Here's the drawing with two shaded views (mm, measured from the low corner). I have some questions. Coordinates: 2 decimals unless noted, no trailing zeros. Write each loop counter-clockwise with the first axis right and the second up, starting at its lowest first coordinate (ties: lowest second). Pieces come first, ordered by that corner, then holes. Notation, with made-up numbers: M -12.75,-17 L 21.25,-17 A35 cw 21.25,15 Z; hole C 66.25,-3 d3. An arc over 180 degrees is marked long. Use one line per item in the form item = value. Start each with the question number.
1. I want a section at A-A, the plane x = 12.5. List the corners of the cut face in (y, z) for me.
2. Thinking about a two-plate mould opening in X: for the marked faces 1, 2 and 3, which applies, released by +X, released by -X, zero draft, split by the parting line, or undercut?
3. I want a section at B-B, the plane y = 18. List the corners of the cut face in (x, z) for me (1 decimal).
4. I want a section at D-D, the plane x = 17.25. List the corners of the cut face in (y, z) for me, plus the area to 3 significant figures.
5. Please list where these lines run through material, in increasing order: line 1 along Y through (x, z) = (10.75, 12); line 2 along X through (y, z) = (15.5, 10.5); line 3 along Y through (x, z) = (10, 7.75). Write a range as [from, to].
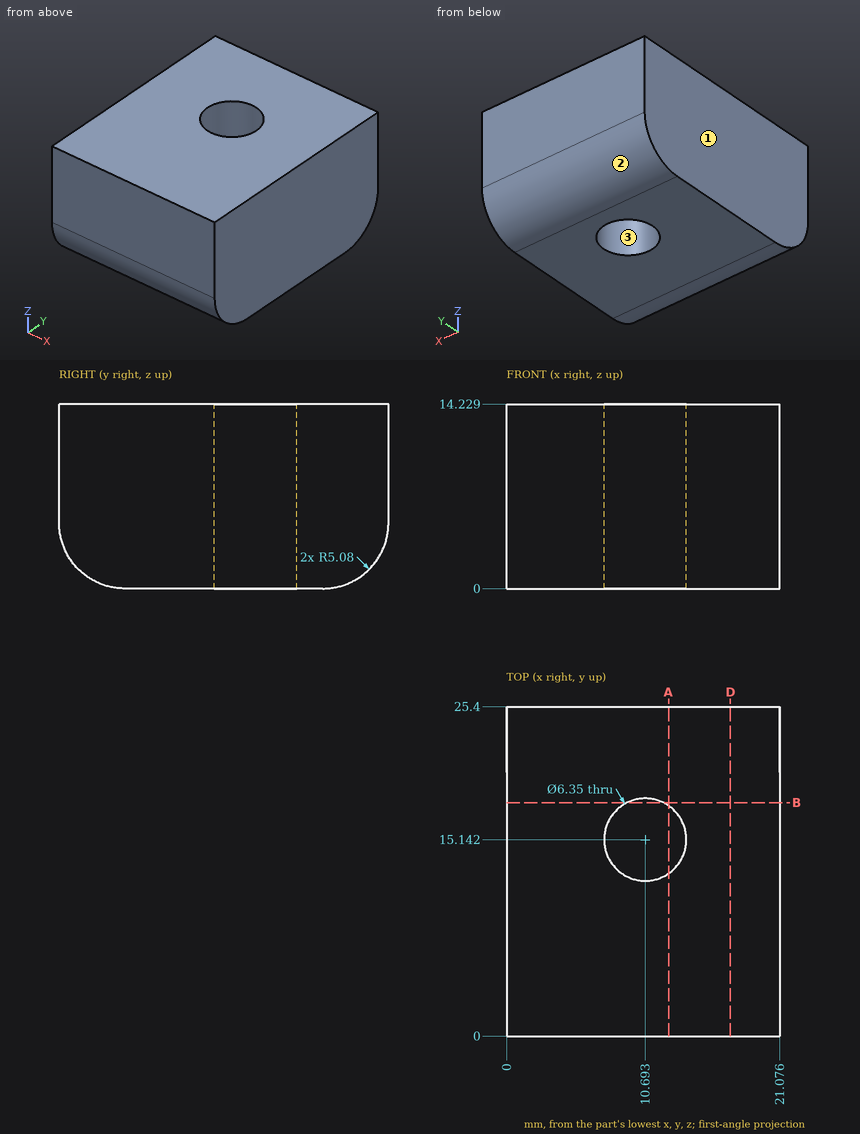
Answer list:
q1.outline = M 0,5.08 A5.08 ccw 5.08,0 L 12.53,0 L 12.53,14.23 L 0,14.23 Z; M 17.75,0 L 20.32,0 A5.08 ccw 25.4,5.08 L 25.4,14.23 L 17.75,14.23 Z
q2.face_1 = released by -X
q2.face_2 = zero draft
q2.face_3 = undercut
q3.outline = M 0,0 L 9.3,0 L 9.3,14.2 L 0,14.2 Z; M 12.1,0 L 21.1,0 L 21.1,14.2 L 12.1,14.2 Z
q4.outline = M 0,5.08 A5.08 ccw 5.08,0 L 20.32,0 A5.08 ccw 25.4,5.08 L 25.4,14.23 L 0,14.23 Z
q4.area = 350 mm²
q5.line_1 = [0, 11.97], [18.32, 25.4]
q5.line_2 = [0, 7.54], [13.85, 21.08]
q5.line_3 = [0, 12.04], [18.24, 25.4]
